Model file for the job. Use its own axes, mm. A direction names the side the tool comes from. Round coordinates to 2 decimals unless told otherwise and drop trailing zeros. Write each loop counter-clockwise with the first axis right and the second up, starting at its lowest first coordinate (ties: lowest second). Pieces come first, ordered by that corner, then holes. Notation, with made-up numbers: (-5, 70) - (43, 70) arc R21 ccw to (43, 86) - close; hole circle Ø2 at (-24.75, 17). An arc over 180 degrees is marked (long way). One line per item, written item: value.
Autodesk Inventor part; units mm, degrees
ref_plane "РабПлоскость1" through (0, 14.5, 0) normal (0, 1, 0) x (-1, 0, 0)
ref_plane "РабПлоскость2" through (0, 0, 18.5) normal (0, 0, 1) x (1, 0, 0)
ref_plane "YZ Plane" through (0, 0, 0) normal (1, 0, 0) x (0, 1, 0)
sketch "Эскиз1" plane through (0, 0, 0) normal (0, 0, 1) x (1, 0, 0)
  line L0 (0, 0) -> (-160, 0)
  line L1 (0, 0) -> (0, 15.4226)
  line L2 (0, 15.4226) -> (-1, 16)
  line L3 (-1, 16) -> (-60, 16)
  line L4 (-60, 16) -> (-60, 17.5)
  line L5 (-60, 17.5) -> (-80, 17.5)
  line L6 (-80, 17.5) -> (-80, 20)
  line L7 (-80, 20) -> (-140, 20)
  line L8 (-140, 20) -> (-140, 17.5)
  line L9 (-140, 17.5) -> (-160, 17.5)
  line L10 (-160, 17.5) -> (-160, 0)
  dimension "d0" = 160
  dimension "d1" = 32
  dimension "d2" = 30
  dimension "d3" = 1
  dimension "d4" = 60
  dimension "d5" = 35
  dimension "d6" = 20
  dimension "d7" = 40
revolve "Вращение1" add sketch "Эскиз1" angle 360 about axis through (0, 0, 0) along (-1, 0, 0)
ref_plane "РабПлоскость1" through (0, 14.5, 0) normal (0, 1, 0) x (-1, 0, 0)
ref_plane "РабПлоскость2" through (0, 0, 18.5) normal (0, 0, 1) x (1, 0, 0)
sketch "Эскиз3" plane through (0, 14.5, 0) normal (0, 1, 0) x (-1, 0, 0)
  line L0 (0, 15.4226) -> (0, -15.4226)
  line L1 (80, 20) -> (80, -20)
  line L2 (140, 20) -> (140, -20)
  line L3 (44, 0) -> (16, 0) construction
  line L4 (40, 4) -> (20, 4)
  line L5 (20, -4) -> (40, -4)
  arc A0 (40, -4) -> (40, 4) centre (40, 0) ccw
  arc A1 (20, 4) -> (20, -4) centre (20, 0) ccw
  point P0 (0, 0)
  point P1 (30, 0)
  point P2 (80, 0)
  dimension "d11" = 20
  dimension "d12" = 8
  dimension "d13" = 50
extrude "Выдавливание1" cut sketch "Эскиз3" along normal through all
sketch "Эскиз4" plane through (0, 0, 18.5) normal (0, 0, 1) x (1, 0, 0)
  line L0 (-124, 0) -> (-96, 0) construction
  line L1 (-120, -4) -> (-100, -4)
  line L2 (-100, 4) -> (-120, 4)
  arc A0 (-120, 4) -> (-120, -4) centre (-120, 0) ccw
  arc A1 (-100, -4) -> (-100, 4) centre (-100, 0) ccw
  line L3 (-80, -17.5) -> (-80, 17.5)
  point P0 (0, 0)
  point P1 (-110, 0)
  point P2 (-80, 0)
  dimension "d16" = 20
  dimension "d17" = 8
  dimension "d18" = 30
extrude "Выдавливание2" cut sketch "Эскиз4" along normal through all
sketch "Эскиз6" plane through (0, 0, 18.5) normal (0, 0, 1) x (1, 0, 0)
  circle A0 centre (-8, 0) radius 2.5
  point P0 (0, 0)
  dimension "d21" = 5
  dimension "d22" = 8
extrude "Выдавливание3" cut sketch "Эскиз6" against normal through all
properties part number "Shaft2"
1. Mould opens along X. For faces 5 (the face through (-80, 0, 18)), 6 (the face through (-16, 15, 0)), 7 (the face through (-160, 0, 0)), 8 (the face through (-150.14, -13.887, 10.648)) say: released by +X, released by -X, zero draft, split by the parting line, or undercut.
Report:
face 5: released by +X
face 6: undercut
face 7: released by -X
face 8: zero draft
2. Drop flat-ended pins along their axis: pin 1 (1 mm diameter, centred on x = -53, y = -11.5, fed in from +Z); pin 2 (4 mm diameter, centred on x = -111, y = -5, fed in from -Z); pin 3 (6.5 mm diameter, centred on x = -34.5, z = -0.5, fed in from +Y); pin 4 (4.5 mm diameter, centred on x = -8, y = 0, fed in from +Z). Give the stop position or say it passes through.
Report:
pin 1: z = 11.62
pin 2: z = -19.77
pin 3: y = 14.5
pin 4: through
3. Band-saw the part on B-B on z = 0. Write the cut outline in (x, y).
Report:
outline: (-160, -17.5) - (-140, -17.5) - (-140, -20) - (-80, -20) - (-80, -17.5) - (-60, -17.5) - (-60, -16) - (-1, -16) - (0, -15.42) - (0, 15.42) - (-1, 16) - (-16, 16) - (-16, 14.5) - (-44, 14.5) - (-44, 16) - (-60, 16) - (-60, 17.5) - (-80, 17.5) - (-80, 20) - (-140, 20) - (-140, 17.5) - (-160, 17.5) - close; hole circle Ø5 at (-8, 0)
4. Band-saw the part on C-C on x = -48. Write the cut outline in (y, z).
Report:
outline: circle Ø32 at (0, 0)
5. Wall check: probe 1 along X at (y, z) = (0, 3.5); probe 2 along Y at (x, z) = (-8, 1); probe 3 along Y at (x, z) = (-8, -3). Give the ranges that are in metal, low to high. Write a range as [from, to].
Report:
probe 1: [-160, -10.5], [-5.5, 0]
probe 2: [-15.97, -2.5], [2.5, 15.97]
probe 3: [-15.72, -2.5], [2.5, 15.72]
6. Band-saw the part on D-D on x = -8. Write the cut outline in (y, z).
Report:
outline: (-2.5, -15.8) - (-2.5, 15.8) arc R16 ccw to start; (2.5, -15.8) arc R16 ccw to (2.5, 15.8) - close
7. Band-saw the part on A-A on y = 0. Write the cut outline in (x, z).
Report:
outline: (-160, -17.5) - (-140, -17.5) - (-140, -20) - (-80, -20) - (-80, -17.5) - (-60, -17.5) - (-60, -16) - (-10.5, -16) - (-10.5, 16) - (-60, 16) - (-60, 17.5) - (-80, 17.5) - (-80, 20) - (-96, 20) - (-96, 18.5) - (-124, 18.5) - (-124, 20) - (-140, 20) - (-140, 17.5) - (-160, 17.5) - close; (-5.5, -16) - (-1, -16) - (0, -15.42) - (0, 15.42) - (-1, 16) - (-5.5, 16) - close
8. Tool access for faces 1 (the face through (-60, 7.7, 14.2)), 2 (the face through (-30, 14.5, 0)), 3 (the face through (-140, 0, 18)), 4 (the face through (-110, 0, 18.5)): list every direction of +Z, -Z, +X, -X, +Y, -Y with a clear straight run to the whole face (end or side of a thin tool).
Report:
face 1: +X
face 2: +Y
face 3: -X
face 4: +Z
